Input: dimensioned drawing with shaded views. Units: mm. Origin: part minimum x, y, z. Give positions to 0.01 mm unless a question says otherwise; leave off trailing zeros. Order: outer loops, then holes, each group sorted by start corner. A loop starts at its lowest first (then second) coordinate and runs counter-clockwise, first axis right, second up.
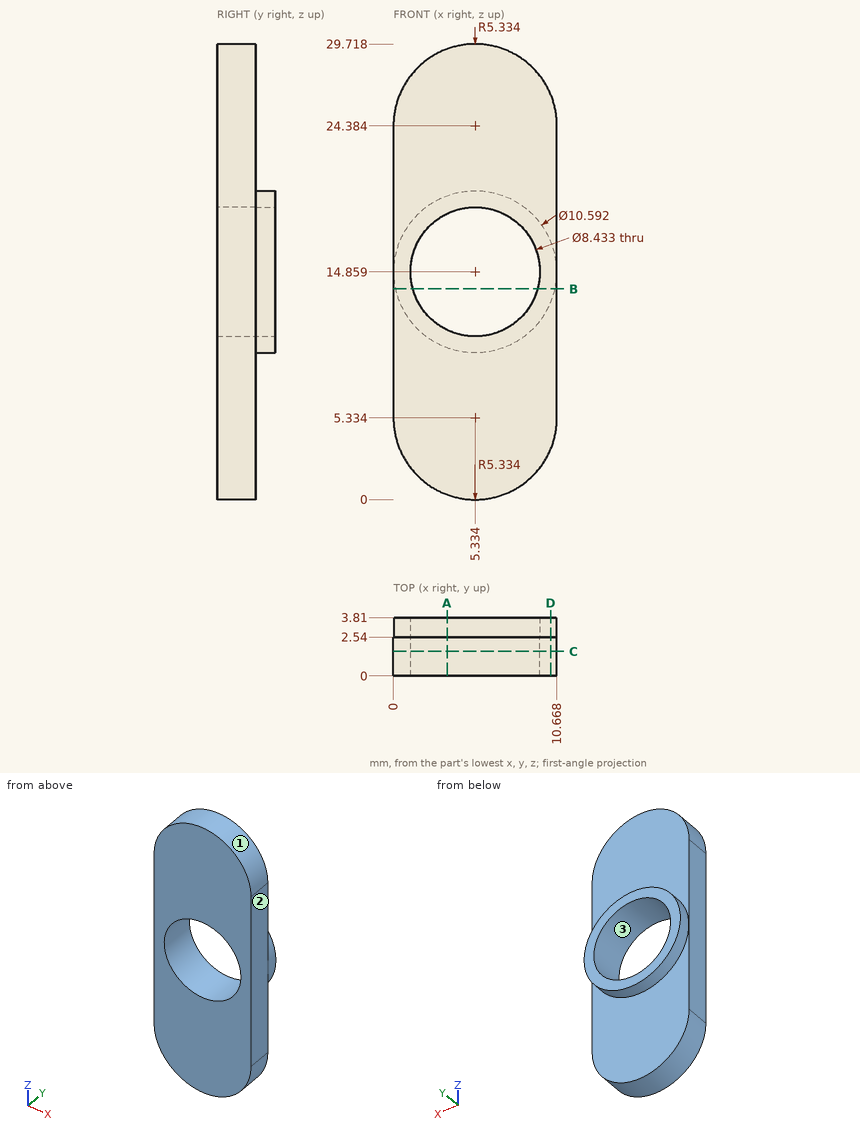
1) Cut plane D-D (x = 10.25). Return the cut outline in (y, z), then the cut area to 3 significant figures.
2) First-contact query: P1, Ø2, axis at x = 5.5, y = 2.5, coming from the -Z side; P2, Ø1, axis at x = 2.5, y = 2.5, coming from the -Z side; P3, Ø1, axis at x = 1, y = 3.5, coming from the +Z side; P4, Ø1.5, axis at x = 2.5, z = 4.5, coming from the +Y side. Flat tips, straight axial feed; report the tip coordinate or a pass-through.
3) Cut plane B-B (z = 13.75). Return the cut outline in (x, y).
4) Pull-direction query (Z, two-part tool) for the marked faces 1, 2 and 3; classes: pulls with the +Z half, pulls with the -Z half, needs draft (parallel to the pull), parting line crosses it, or undercut.
5) Line query: probe 1 along Z at (x, y) = (5.5, 0.3) (1 decimal); probe 2 along X at (y, z) = (2.25, 25); probe 3 along Z at (x, y) = (3, 2.2). Output: solid intervals per line, ascending.
6) Cut plane A-A (x = 3.5). Return the cut outline in (y, z) (1 decimal), then the cut area to 3 significant figures.
7) Cut plane C-C (y = 1.6). Return the cut outline in (x, z).
Geometry says:
1. outline: (0, 3.26) - (2.54, 3.26) - (2.54, 12.89) - (3.81, 12.89) - (3.81, 16.83) - (2.54, 16.83) - (2.54, 26.45) - (0, 26.45) - close
1. area: 63.9 mm2
2. P1: stops at z = 0
2. P2: stops at z = 0.54
2. P3: stops at z = 18.51
2. P4: stops at y = 2.54
3. outline: (0, 0) - (1.27, 0) - (1.27, 3.81) - (0.16, 3.81) - (0.16, 2.54) - (0, 2.54) - close; (9.4, 0) - (10.67, 0) - (10.67, 2.54) - (10.51, 2.54) - (10.51, 3.81) - (9.4, 3.81) - close
4. face 1: pulls with the +Z half
4. face 2: needs draft
4. face 3: undercut
5. probe 1: z = 0 to 10.6, 19.1 to 29.7
5. probe 2: x = 0.04 to 10.63
5. probe 3: z = 0.54 to 11.35, 18.37 to 29.18
6. outline: (0, 0.3) - (2.5, 0.3) - (2.5, 9.9) - (3.8, 9.9) - (3.8, 11.1) - (0, 11.1) - close; (0, 18.7) - (3.8, 18.7) - (3.8, 19.8) - (2.5, 19.8) - (2.5, 29.4) - (0, 29.4) - close
6. area: 57.5 mm2
7. outline: (0, 5.33) arc R5.33 ccw to (10.67, 5.33) - (10.67, 24.38) arc R5.33 ccw to (0, 24.38) - close; hole circle Ø8.43 at (5.33, 14.86)
